Read the model definition and answer for the solid it produces. Units are mm, in the model's axes. A direction names the side the tool comes from. Give positions to 0.01 mm unless a question says otherwise; leave off trailing zeros. Order: outer loops, then holes, each group sorted by start corner. A loop starts at its lowest first (then second) coordinate and runs counter-clockwise, first axis right, second up. Notation, with made-up numbers: (70, 12.5) -> (122, 12.5) arc R27 ccw to (122, 35.5) -> close; hole circle Ø3 at (78.25, -24.5). An arc over 180 degrees is marked (long way). Answer as CSV lines item,"result". Start each with the question number.
1) Straight lines are drawn through the part: L1, parallel to Y at x = -24.5, z = 38; L2, parallel to Y at x = 5, z = 41; L3, parallel to Z at x = -31, y = 2.5. For each, find the intervals that lie inside material, in ascending order. Write a range as from..to.
2) Find section A-A (y = -4). Determine the outline of the cut face in (x, z), and give its area (3 significant figures).
3) Find section C-C (z = 87). Determine the outline of the cut face in (x, y), and give its area (3 significant figures).
4) Find section B-B (x = 22). Determine the outline of the cut face in (y, z) (3 decimals).
5) For faces 1 (the face through (0.533, -9.724, 65.401)), 2 (the face through (-28, -44.863, 32)), 3 (the face through (-28.442, -37.242, 36.395)), determine the directions among +Z, -Z, +X, -X, +Y, -Y from which every point of the face is accessible in a straight line to the end or side of a thin tool.
6) Flat-ended cylindrical pins translate along their axes: pin 1 Ø12 at (x, y) = (-11, 15.5) entering from +Z; pin 2 Ø5 at (x, z) = (-7, 63) entering from -Y; pin 3 Ø8 at (x, y) = (26, -40.5) entering from +Z. Find the tip coordinate at first contact, or state that the pin passes through.
7) The mould has two halves that part along Y. Classify faces 4 (the face through (28.708, -37.242, 36.395)), 5 (the face through (0.53, 16.13, 10.5)), 6 (the face through (-1, -5, 101.6)): +Y half, -Y half, draft (parallel to the pull), parting line (faces both ways), or undercut.
8) Find section D-D (x = -14). Determine the outline of the cut face in (y, z) (3 decimals), and give its area (3 significant figures).
```python
from build123d import *

# Parameters (mm, degrees)
F0_W     = 76.2
F0_H     = 101.6
F1_DEPTH = 101.6
F3_DEPTH = 76.201
F4_W     = 38.1
F4_H     = 9.0885387092
F5_DEPTH = 25.4
F7_DEPTH = 19.05


with BuildPart() as f1:
    # F0 (on Top) → F1 (new body)
    with BuildSketch(Plane.XY):
        Rectangle(F0_W, F0_H)
    extrude(amount=F1_DEPTH)

    # F2 (on face) → F3 (cut, through all)
    with BuildSketch(Plane.YZ.offset(38.1)):
        with BuildLine():
            Line((50.8, 101.6), (0, 101.6))
            Line((0, 101.6), (-19.7247579018, 28.1743642605))
            ThreePointArc((-19.7247579018, 28.1743642605), (-18.6322824559, 20.7020087833), (-12.4441793676, 16.3733855441))
            Line((-12.4441793676, 16.3733855441), (45.5164201772, 4.4562514699))
            ThreePointArc((45.5164201772, 4.4562514699), (45.6671065402, 4.4046156558), (45.799921858, 4.316679721))
            Line((45.799921858, 4.316679721), (49.5238091926, 1.1017641769))
            ThreePointArc((49.5238091926, 1.1017641769), (49.7017678057, 0.4084810434), (49.114014449, 0))
            Line((49.114014449, 0), (50.8, 0))
            Line((50.8, 0), (50.8, 101.6))
        make_face()
        with BuildLine():
            Line((-29.1485272072, 29.8082903279), (-9.8627004197, 101.6))
            Line((-9.8627004197, 101.6), (-50.8, 101.6))
            Line((-50.8, 101.6), (-50.8, 0))
            Line((-50.8, 0), (-49.3153884285, 0))
            ThreePointArc((-49.3153884285, 0), (-49.8930613229, 0.38308634), (-49.7649416709, 1.0642959051))
            Line((-49.7649416709, 1.0642959051), (-45.0471924847, 5.9153086442))
            ThreePointArc((-45.0471924847, 5.9153086442), (-44.8416453701, 6.0557781013), (-44.5976392423, 6.1051976748))
            Line((-44.5976392423, 6.1051976748), (-35.9854393765, 6.1051976748))
            ThreePointArc((-35.9854393765, 6.1051976748), (-35.6522704088, 6.2010242938), (-35.4209251987, 6.4592174303))
            Line((-35.4209251987, 6.4592174303), (-31.6196714319, 20.6094278319))
            Line((-31.6196714319, 20.6094278319), (-32.3972816474, 20.8183218113))
            Line((-32.3972816474, 20.8183218113), (-44.3981189181, 24.042176905))
            ThreePointArc((-44.3981189181, 24.042176905), (-44.7330556249, 24.2662072787), (-44.8625199497, 24.6477976277))
            Line((-44.8625199497, 24.6477976277), (-44.8625199497, 40.5587139142))
            ThreePointArc((-44.8625199497, 40.5587139142), (-44.6788488183, 41.0021352507), (-44.2354274818, 41.1858063821))
            Line((-44.2354274818, 41.1858063821), (-36.772603948, 41.1858063821))
            ThreePointArc((-36.772603948, 41.1858063821), (-36.2749758049, 40.9403042633), (-36.1669832252, 40.396022478))
            Line((-36.1669832252, 40.396022478), (-38.3473897032, 32.2794345527))
            Line((-38.3473897032, 32.2794345527), (-29.1485272072, 29.8082903279))
        make_face()
    extrude(amount=-F3_DEPTH, mode=Mode.SUBTRACT)

    # F4 (on face) → F5 (cut)
    with BuildSketch(Plane(origin=(0, -34.6552022965, 9.3096296471), x_dir=(1, 0, 0), z_dir=(0, -0.9657598421, 0.2594377139))):
        with Locations((0, 25.7696918533)):
            Rectangle(F4_W, F4_H)
    extrude(amount=F5_DEPTH, mode=Mode.SUBTRACT)

    # F6 (on face) → F7 (cut)
    with BuildSketch(Plane(origin=(0, 5.5066750893, 20.4986606809), x_dir=(1, 0, 0), z_dir=(0, 0.2594377139, 0.9657598421))):
        Polygon((-19.05, -45.4088717305), (-19.05, -52.1549901364), (19.05, -52.1549901364), (19.05, -45.4088717305), (19.05, -35.8838717305), (-19.05, -35.8838717305), align=None)
    extrude(amount=-F7_DEPTH, mode=Mode.SUBTRACT)


solid = f1.part
```
Findings below:
1,L1,"-44.86..-36.81, -26.95..-17.09"
1,L2,"-26.14..-16.28"
1,L3,"0..13.3"
2,outline,"(-38.1, 0) -> (38.1, 0) -> (38.1, 14.64) -> (-38.1, 14.64) -> close; (-38.1, 86.71) -> (38.1, 86.71) -> (38.1, 101.6) -> (-38.1, 101.6) -> close"
2,area,"2,250 mm²"
3,outline,"(-38.1, -13.78) -> (38.1, -13.78) -> (38.1, -3.92) -> (-38.1, -3.92) -> close"
3,area,"752 mm²"
4,outline,"(-49.765, 1.064) arc R0.627 ccw to (-49.315, 0) -> (49.114, 0) arc R0.627 ccw to (49.524, 1.102) -> (45.8, 4.317) arc R0.627 ccw to (45.516, 4.456) -> (-12.444, 16.373) arc R9.525 cw to (-19.725, 28.174) -> (0, 101.6) -> (-9.863, 101.6) -> (-29.149, 29.808) -> (-38.347, 32.279) -> (-36.167, 40.396) arc R0.627 ccw to (-36.773, 41.186) -> (-44.235, 41.186) arc R0.627 ccw to (-44.863, 40.559) -> (-44.863, 24.648) arc R0.627 ccw to (-44.398, 24.042) -> (-31.62, 20.609) -> (-35.421, 6.459) arc R0.627 cw to (-35.985, 6.105) -> (-44.598, 6.105) arc R0.627 ccw to (-45.047, 5.915) -> close"
5,face 1,"+X, -X, +Y"
5,face 2,"+Z, +X, -X, -Y"
5,face 3,"+X, -X"
6,pin 1,"z = 11.86"
6,pin 2,"y = -20.9"
6,pin 3,"z = 41.19"
7,face 4,"undercut"
7,face 5,"+Y half"
7,face 6,"draft"
8,outline,"(-49.765, 1.064) arc R0.627 ccw to (-49.315, 0) -> (49.114, 0) arc R0.627 ccw to (49.524, 1.102) -> (45.8, 4.317) arc R0.627 ccw to (45.516, 4.456) -> (-12.444, 16.373) arc R9.525 cw to (-19.725, 28.174) -> (0, 101.6) -> (-9.863, 101.6) -> (-35.421, 6.459) arc R0.627 cw to (-35.985, 6.105) -> (-44.598, 6.105) arc R0.627 ccw to (-45.047, 5.915) -> close"
8,area,"1,930 mm²"
